from build123d import *

# Parameters (mm, degrees)
F0_W      = 19.05
F0_H      = 19.05
F1_DEPTH  = 9.525
F2_R      = 2
F3_DEPTH  = 1.6
F4_R      = 2
F5_DEPTH  = 1.6
F6_R      = 2
F7_DEPTH  = 1.6
F8_R      = 2
F9_DEPTH  = 1.6
F10_R     = 2
F11_DEPTH = 1.6
F12_R     = 2
F13_DEPTH = 1.6


with BuildPart() as f1:
    # F0 (on Top) → F1 (new body, symmetric)
    with BuildSketch(Plane.XY):
        Rectangle(F0_W, F0_H)
    extrude(amount=F1_DEPTH, both=True)

    # F2 (on face) → F3 (cut)
    with BuildSketch(Plane.XY.offset(9.525)):
        Circle(F2_R)
    extrude(amount=-F3_DEPTH, mode=Mode.SUBTRACT)

    # F4 (on face) → F5 (cut)
    with BuildSketch(Plane.XZ.offset(9.525)):
        with Locations((-4.525, -4.525)):
            Circle(F4_R)
        with Locations((4.525, 4.525)):
            Circle(F4_R)
    extrude(amount=-F5_DEPTH, mode=Mode.SUBTRACT)

    # F6 (on face) → F7 (cut)
    with BuildSketch(Plane(origin=(0, 0, -9.525), x_dir=(1, 0, 0), z_dir=(0, 0, -1))):
        with Locations((-4.525, -4.525)):
            Circle(F6_R)
        with Locations((-4.525, 4.525)):
            Circle(F6_R)
        with Locations((4.525, -4.525)):
            Circle(F6_R)
        with Locations((4.525, 4.525)):
            Circle(F6_R)
        with Locations((-4.525, 0)):
            Circle(F6_R)
        with Locations((4.525, 0)):
            Circle(F6_R)
    extrude(amount=-F7_DEPTH, mode=Mode.SUBTRACT)

    # F8 (on face) → F9 (cut)
    with BuildSketch(Plane(origin=(0, 9.525, 0), x_dir=(-1, 0, 0), z_dir=(0, 1, 0))):
        with Locations((-4.525, -4.525)):
            Circle(F8_R)
        Circle(F8_R)
        with Locations((-4.525, 4.525)):
            Circle(F8_R)
        with Locations((4.525, -4.525)):
            Circle(F8_R)
        with Locations((4.525, 4.525)):
            Circle(F8_R)
    extrude(amount=-F9_DEPTH, mode=Mode.SUBTRACT)

    # F10 (on face) → F11 (cut)
    with BuildSketch(Plane.YZ.offset(9.525)):
        with Locations((-4.525, -4.525)):
            Circle(F10_R)
        Circle(F10_R)
        with Locations((4.525, 4.525)):
            Circle(F10_R)
    extrude(amount=-F11_DEPTH, mode=Mode.SUBTRACT)

    # F12 (on face) → F13 (cut)
    with BuildSketch(Plane(origin=(-9.525, 0, 0), x_dir=(0, -1, 0), z_dir=(-1, 0, 0))):
        with Locations((-4.525, -4.525)):
            Circle(F12_R)
        with Locations((-4.525, 4.525)):
            Circle(F12_R)
        with Locations((4.525, -4.525)):
            Circle(F12_R)
        with Locations((4.525, 4.525)):
            Circle(F12_R)
    extrude(amount=-F13_DEPTH, mode=Mode.SUBTRACT)


solid = f1.part
Verification items for the finished model (mm, model axes). A direction names the side the tool comes from. Coordinates: 2 decimals unless noted, no trailing zeros. Order: outer loops, then holes, each group sorted by start corner. A loop starts at its lowest first (then second) coordinate and runs counter-clockwise, first axis right, second up.
Item 1: Section check A-A, the plane x = 0. Enter the section's corners in (y, z) (3 decimals), then the cut area to 3 significant figures.
Filled in:
outline: (-9.525, -9.525) - (9.525, -9.525) - (9.525, -2) - (7.925, -2) - (7.925, 2) - (9.525, 2) - (9.525, 9.525) - (2, 9.525) - (2, 7.925) - (-2, 7.925) - (-2, 9.525) - (-9.525, 9.525) - close
area: 350 mm2
Item 2: Section check D-D, the plane z = -3.25. Enter the section's corners in (x, y) (3 decimals), then the cut area to 3 significant figures.
Filled in:
outline: (-9.525, -9.525) - (-6.066, -9.525) - (-6.066, -7.925) - (-2.984, -7.925) - (-2.984, -9.525) - (9.525, -9.525) - (9.525, -6.066) - (7.925, -6.066) - (7.925, -2.984) - (9.525, -2.984) - (9.525, 9.525) - (6.066, 9.525) - (6.066, 7.925) - (2.984, 7.925) - (2.984, 9.525) - (-2.984, 9.525) - (-2.984, 7.925) - (-6.066, 7.925) - (-6.066, 9.525) - (-9.525, 9.525) - (-9.525, 6.066) - (-7.925, 6.066) - (-7.925, 2.984) - (-9.525, 2.984) - (-9.525, -2.984) - (-7.925, -2.984) - (-7.925, -6.066) - (-9.525, -6.066) - close
area: 333 mm2
Item 3: Depth check by flat-ended pin: pin 1 (2.5 mm diameter, centred on x = -4.525, z = 4.525, fed in from +Y) (3 decimals); pin 2 (1.2 mm diameter, centred on y = -5.5, z = 4, fed in from -X) (3 decimals); pin 3 (2 mm diameter, centred on y = -5, z = -5, fed in from +X) (3 decimals). Enter the tip coordinate at first touch or a pass-through.
Filled in:
pin 1: stops at y = 7.925
pin 2: stops at x = -7.925
pin 3: stops at x = 7.925
Item 4: Access from +Z, -Z, +X, -X, +Y, -Y to the whole of each face (thin tool, end or side, straight path). Record for faces 1 (the face through (-5, 4, -7.925)), 2 (the face through (-8.7, 3.6, -6.3)), 3 (the face through (3.6, 8.7, -6.3)), 4 (the face through (-5, -7.925, -4)).
Filled in:
face 1: -Z
face 2: -X
face 3: +Y
face 4: -Y
Item 5: Section check B-B, the plane y = 0. Enter the section's corners in (x, z) (3 decimals).
Filled in:
outline: (-9.525, -9.525) - (-6.525, -9.525) - (-6.525, -7.925) - (-2.525, -7.925) - (-2.525, -9.525) - (2.525, -9.525) - (2.525, -7.925) - (6.525, -7.925) - (6.525, -9.525) - (9.525, -9.525) - (9.525, -2) - (7.925, -2) - (7.925, 2) - (9.525, 2) - (9.525, 9.525) - (2, 9.525) - (2, 7.925) - (-2, 7.925) - (-2, 9.525) - (-9.525, 9.525) - close
Item 6: Material ranges on L1, parallel to X at y = 0, z = -8.25 (3 decimals); L2, parallel to Z at x = -8, y = 3 (3 decimals); L3, parallel to Z at x = -4.75, y = 8.25 (3 decimals), recorded low to high.
Filled in:
L1: x = -9.525 to -6.525, -2.525 to 2.525, 6.525 to 9.525
L2: z = -9.525 to -5.819, -3.231 to 3.231, 5.819 to 9.525
L3: z = -9.525 to -6.512, -2.538 to 2.538, 6.512 to 9.525
Item 7: Release check for a two-part mould opening along Z. For faces 5 (the face through (-8.74, 3.45, 6.21)), 6 (the face through (4, 4, -7.925)), 7 (the face through (2.94, 1.22, -8.74)) record: +Z half, -Z half, draft (parallel to the pull), parting line (faces both ways), or undercut.
Filled in:
face 5: undercut
face 6: -Z half
face 7: draft
